Input: part model. Units: mm. Frame: model coordinates. Coordinates: 2 decimals unless noted, no trailing zeros. Loops run counter-clockwise (first coordinate to the right, second up) from the corner with the lowest first, then second, coordinate; pieces in that order, holes last.
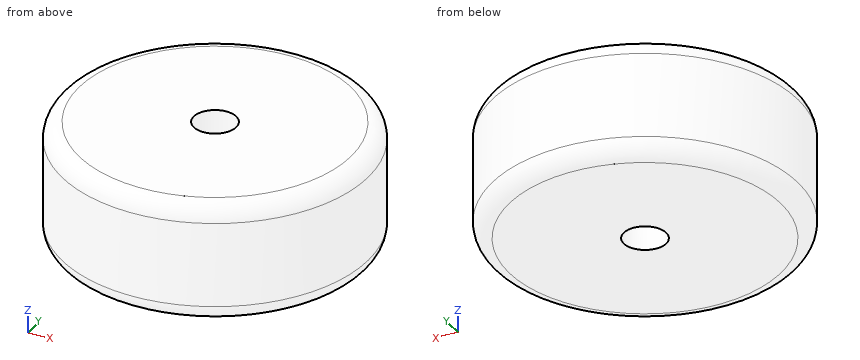
```python
from build123d import *

# Parameters (mm, degrees)
SKETCH1_R           = 18
BOSS_EXTRUDE1_DEPTH = 7
FILLET2_R           = 2
CUT_EXTRUDE1_REACH  = 16
SKETCH2_R           = 2.5


with BuildPart() as part:
    # Sketch1 → Boss-Extrude1 (new body)
    with BuildSketch(Plane.XY):
        Circle(SKETCH1_R)
    boss_extrude1 = extrude(amount=BOSS_EXTRUDE1_DEPTH)

    # Mirror1: Boss-Extrude1 across plane
    add(boss_extrude1.mirror(Plane.XY))

    # Fillet2
    fillet2_edges = [part.edges().sort_by_distance(p)[0] for p in [
        (-18, 0, 7),
        (-18, 0, -7),
    ]]
    fillet(fillet2_edges, radius=FILLET2_R)

    # Sketch2 → Cut-Extrude1 (cut, up to next)
    with BuildSketch(Plane.XY.offset(7), mode=Mode.PRIVATE) as cut_extrude1_sk1:
        Circle(SKETCH2_R)
    cut_extrude1_tool1 = extrude(cut_extrude1_sk1.sketch, amount=-CUT_EXTRUDE1_REACH, mode=Mode.PRIVATE) & part.part
    add(cut_extrude1_tool1.solids().sort_by_distance((0, 0, 7))[0], mode=Mode.SUBTRACT)


solid = part.part
```
Item 1: Section query C-C (z = 2). Output: boundary loops of the cut face in (x, y), then the cut area to 3 significant figures.
Result:
outline: circle Ø36 at (0, 0); hole circle Ø5 at (0, 0)
area: 998 mm2
Item 2: Line query: L1, parallel to Y at x = 0, z = -1.5; L2, parallel to Y at x = 0.5, z = -5.25; L3, parallel to Y at x = 12, z = 3.5. Output: solid intervals per line, ascending.
Result:
L1: y = -18 to -2.5, 2.5 to 18
L2: y = -17.98 to -2.45, 2.45 to 17.98
L3: y = -13.42 to 13.42
Item 3: Contact query for flat-ended pins moving along their axis: P1, Ø1.5, axis at y = 5, z = 5, coming from the +X side; P2, Ø2, axis at x = -7, z = -5.5, coming from the -Y side; P3, Ø5, axis at x = -4.5, z = 2.5, coming from the +Y side. Output: stop coordinate, or through.
Result:
P1: stops at x = 17.49
P2: stops at y = -16.94
P3: stops at y = 17.89
Item 4: Section query A-A (y = 0). Output: boundary loops of the cut face in (x, z), then the cut area to 3 significant figures.
Result:
outline: (-18, -5) arc R2 ccw to (-16, -7) - (-2.5, -7) - (-2.5, 7) - (-16, 7) arc R2 ccw to (-18, 5) - close; (2.5, -7) - (16, -7) arc R2 ccw to (18, -5) - (18, 5) arc R2 ccw to (16, 7) - (2.5, 7) - close
area: 431 mm2
